Geometry: see drawing. Coordinates: mm, zero at the bounding-box minimum. Coordinates: 2 decimals unless noted, no trailing zeros. Loops run counter-clockwise (first coordinate to the right, second up) from the corner with the lowest first, then second, coordinate; pieces in that order, holes last. Notation, with made-up numbers: (88, -8.75) - (101, -8.75) arc R11 ccw to (101, -2.75) - close; hole circle Ø7 at (89.5, 30.5). An arc over 180 degrees is marked (long way). Use one line per item in the form item = value.
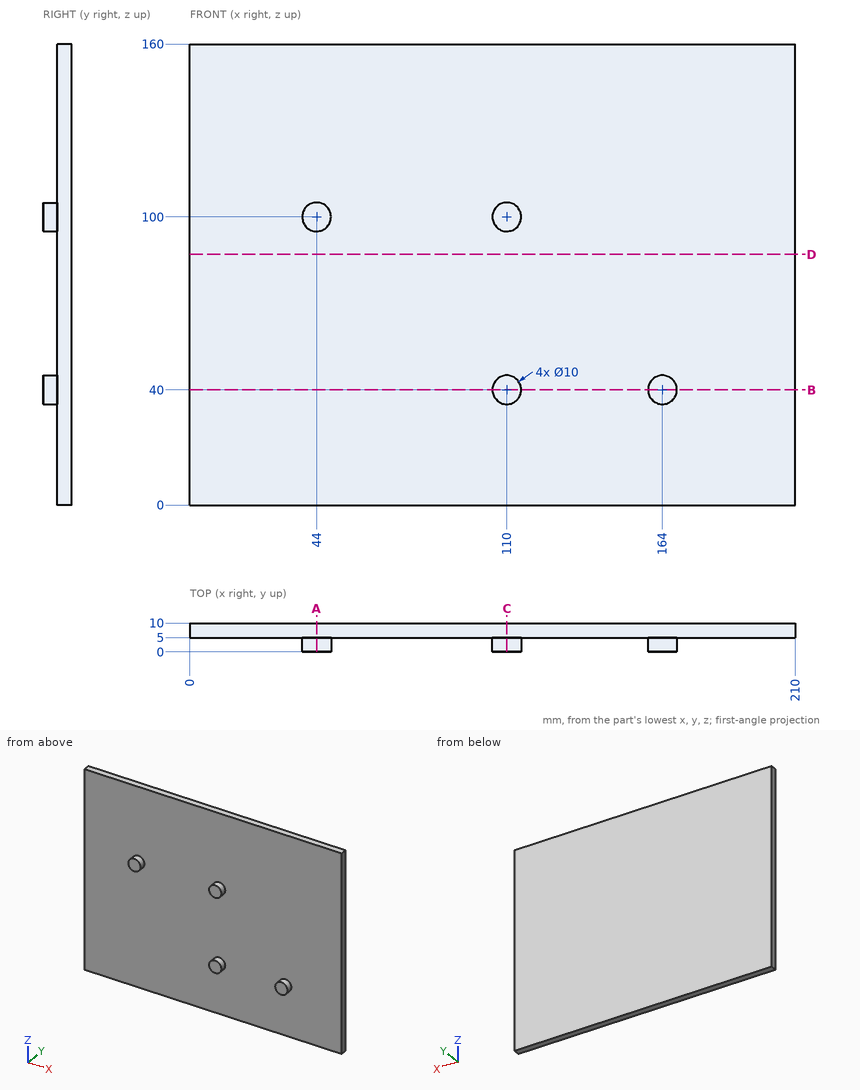
Q1. Cut plane A-A, the plane x = 44. Return loops of the section in (y, z).
Check values:
outline = (0, 95) - (5, 95) - (5, 0) - (10, 0) - (10, 160) - (5, 160) - (5, 105) - (0, 105) - close
Q2. Cut plane B-B, the plane z = 40. Return loops of the section in (x, y), then the cut area to 3 significant figures.
Check values:
outline = (0, 5) - (105, 5) - (105, 0) - (115, 0) - (115, 5) - (159, 5) - (159, 0) - (169, 0) - (169, 5) - (210, 5) - (210, 10) - (0, 10) - close
area = 1,150 mm²
Q3. Ray query, line 1 along Y through (x, z) = (41, 151.5). Return the intervals inside material, ascending. Write a range as [from, to].
Check values:
line_1 = [5, 10]
Q4. First-contact query: P1, Ø1, axis at x = 47, y = 2, coming from the -Z side; P2, Ø6, axis at x = 25, z = 77, coming from the -Y side. Flat tips, straight axial feed; report the tip coordinate or a pass-through.
Check values:
P1 = 95.67
P2 = 5
Q5. Cut plane C-C, the plane x = 110. Return loops of the section in (y, z).
Check values:
outline = (0, 35) - (5, 35) - (5, 0) - (10, 0) - (10, 160) - (5, 160) - (5, 105) - (0, 105) - (0, 95) - (5, 95) - (5, 45) - (0, 45) - close
Q6. Cut plane D-D, the plane z = 87. Return loops of the section in (x, y), then the cut area to 3 significant figures.
Check values:
outline = (0, 5) - (210, 5) - (210, 10) - (0, 10) - close
area = 1,050 mm²
